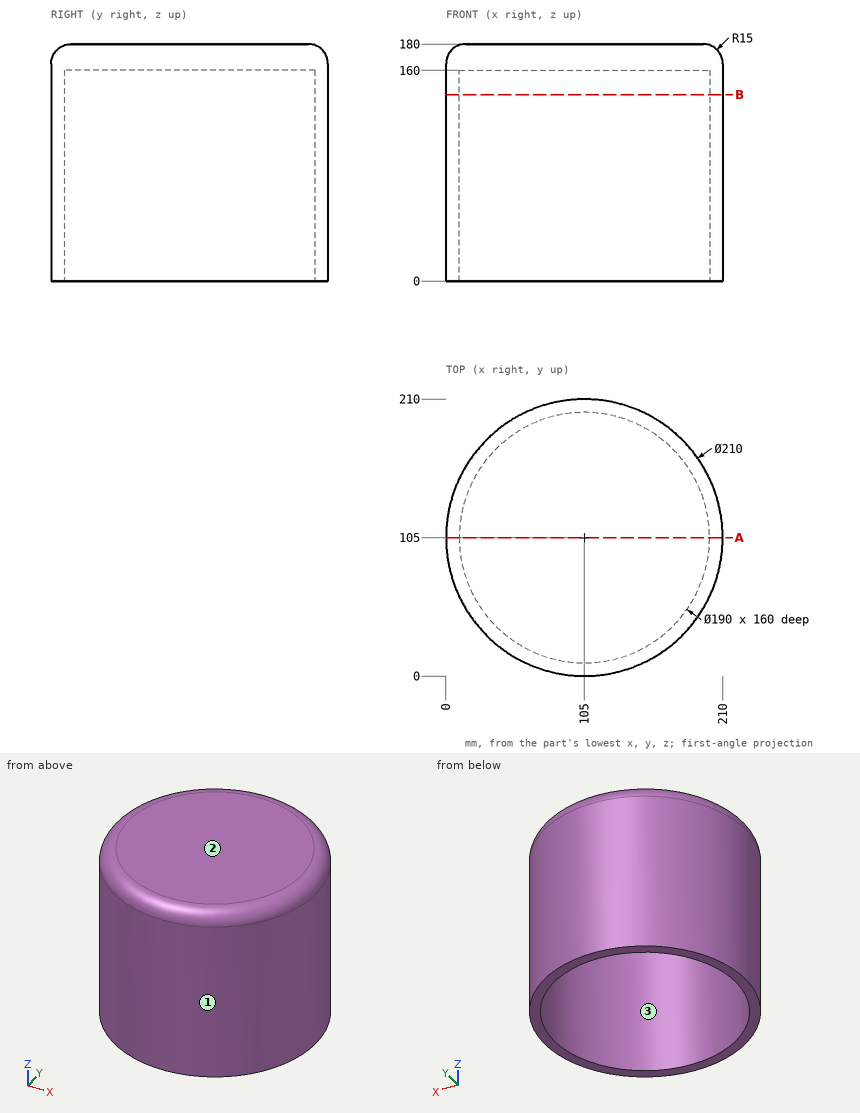
The drawing under review shows one solid part. Ordinate dimensions are in mm from its lowest x, y, z. Round coordinates to 2 decimals unless told otherwise and drop trailing zeros. Write each loop counter-clockwise with the first axis right and the second up, starting at its lowest first coordinate (ties: lowest second). Pieces come first, ordered by that corner, then holes. Notation, with made-up numbers: (42.5, -39) - (79.5, -39) arc R18 cw to (79.5, -11) - close; hole circle Ø10 at (-21.75, 70). An arc over 180 degrees is marked (long way). Use a Markdown table: item, result. Add a question column.
1. We need section A-A (y = 105). State the section outline as (x, z) points, then the cut area to 3 significant figures.
2. Mouldability with a two-part tool opening along X and no side actions: class the marked faces 1, 2 and 3 as +X half, -X half, draft (parallel to the pull), parting line (faces both ways), or undercut.
3. Wall thickness on probe 1 along X at (y, z) = (103.5, 104.5); probe 2 along Y at (x, z) = (105, 92); probe 3 along Z at (x, y) = (100, 110.5): over which ranges is each line inside the solid? List them lowest first.
4. Clearance check with flat-ended pins moving along their axes: pin 1 (12 mm diameter, centred on x = 130, z = 130.5, fed in from +Y); pin 2 (5 mm diameter, centred on x = 22.5, z = 152.5, fed in from +Y); pin 3 (1 mm diameter, centred on y = 53.5, z = 42.5, fed in from -X). State where each tip first meets the part, or that it passes through.
5. We need section B-B (z = 141.5). State the section outline as (x, y) points.
Output:
| question | item | result |
|---|---|---|
| 1 | outline | (0, 0) - (10, 0) - (10, 160) - (200, 160) - (200, 0) - (210, 0) - (210, 165) arc R15 ccw to (195, 180) - (15, 180) arc R15 ccw to (0, 165) - close |
| 1 | area | 7,300 mm2 |
| 2 | face 1 | parting line |
| 2 | face 2 | draft |
| 2 | face 3 | undercut |
| 3 | probe 1 | x = 0.01 to 10.01, 199.99 to 209.99 |
| 3 | probe 2 | y = 0 to 10, 200 to 210 |
| 3 | probe 3 | z = 160 to 180 |
| 4 | pin 1 | stops at y = 208.27 |
| 4 | pin 2 | stops at y = 173.01 |
| 4 | pin 3 | stops at x = 13.22 |
| 5 | outline | circle Ø210 at (105, 105); hole circle Ø190 at (105, 105) |
